CAD build for the part. Positions are in the model's coordinates, mm. Round coordinates to 2 decimals unless told otherwise and drop trailing zeros. Answer as a JSON object with one key per item and string values.
```python
from build123d import *


# Not quite as in the source:
# - ends of sketch curves that miss each other by under 0.0002 mm in the source are joined


with BuildPart() as f1:
    # F0 (on Front) → F1 (revolve)
    with BuildSketch(Plane.XZ):
        with BuildLine():
            Line((0.96, 0), (0.01, 0))
            Line((0.01, 0), (0.01, -0.15))
            Line((0.01, -0.15), (0.96, -0.15))
            ThreePointArc((0.96, -0.15), (1.7476920727, 0.2023696464), (2.61, 0.1700006461))
            ThreePointArc((2.61, 0.1700006461), (2.6139996854, 0.1689036293), (2.6179969666, 0.1677978844))
            ThreePointArc((2.6179969666, 0.1677978844), (3.1597730322, 0.1590424375), (3.64, 0.4100006461))
            ThreePointArc((3.64, 0.4100006461), (3.6431863407, 0.4128835368), (3.646379193, 0.4157592141))
            ThreePointArc((3.646379193, 0.4157592141), (4.4496112836, 0.8443127993), (5.36, 0.8500006461))
            Line((5.36, 0.8500006461), (6.41, 0.8500006461))
            Line((6.41, 0.8500006461), (6.41, 1))
            Line((6.41, 1), (5.36, 1))
            ThreePointArc((5.36, 1), (4.4496112836, 0.9943121532), (3.646379193, 0.565758568))
            ThreePointArc((3.646379193, 0.565758568), (3.6431863407, 0.5628828907), (3.64, 0.56))
            ThreePointArc((3.64, 0.56), (3.1597730322, 0.3090417914), (2.6179969666, 0.3177972383))
            ThreePointArc((2.6179969666, 0.3177972383), (2.6139996854, 0.3189029832), (2.61, 0.32))
            ThreePointArc((2.61, 0.32), (1.7476920727, 0.3523690002), (0.96, 0))
        make_face()
    revolve(axis=Axis((-13.59, 0, 6.1745331623), (0, 0, 1)))


solid = f1.part
```
Item 1: Drop flat-ended pins along their axis: pin 1 Ø8 at (x, y) = (1.5, -15.5) entering from -Z; pin 2 Ø23.5 at (x, y) = (-16.5, -0.5) entering from +Z. Give the stop position or say it passes through.
Worked answers:
{"pin 1": "stops at z = 0.69", "pin 2": "stops at z = 0.1"}
Item 2: Wall check: line 1 along Y through (x, z) = (-13.59, -0.1); line 2 along X through (y, z) = (-9, 0.6); line 3 along Y through (x, z) = (-13.59, -0.05). Give the ranges that are in metal, low to high. Write a range as [from, to].
Worked answers:
{"line 1": "y = [-14.62, -13.6], [13.6, 14.62]", "line 2": "x = [-28.57, -28.34], [1.16, 1.39]", "line 3": "y = [-14.7, -13.6], [13.6, 14.7]"}
Item 3: Two-plate mould, pull along X, no slides. Class faces 1 (the flat face through (-4, -10, 0)), 2 (the flat face through (-31.3, -7.3, 0.85)): released by +X, released by -X, zero draft, split by the parting line, or undercut.
Worked answers:
{"face 1": "undercut", "face 2": "zero draft"}
